Can you work these out from the model? Positions are in its coordinate system, mm. A direction names the side the tool comes from. Coordinates: 2 decimals unless noted, no trailing zeros. Write each loop counter-clockwise with the first axis right and the second up, starting at its lowest first coordinate (ties: lowest second). Pieces come first, ordered by that corner, then holes. Notation, with made-up numbers: (-24.5, -21) - (32.5, -21) arc R22 cw to (32.5, 15) - close; hole circle Ø7 at (-4, 56). An arc over 180 degrees is marked (long way). Use one line per item in the form item = value. Start each with the question number.
(1) If I drill on probe 1 along Z at (x, y) = (-14, 12); probe 2 along Y at (x, z) = (-35, -5.9); probe 3 along Y at (x, z) = (-23, -4), over which ranges is the centre line in solid material (lowest first)? Write a range as from..to.
(2) For pin 1 Ø2.5 at (x, y) = (45.89, 14.18) entering from -Z; pin 2 Ø2.5 at (x, y) = (74.11, 14.18) entering from +Z; pin 3 Ø3 at (y, z) = (2, 3) entering from +X; pin 4 Ø4.5 at (x, z) = (34, 1) entering from -Y, each with a flat end and sliding along its axis, tell me the tip position at first contact or that it passes through.
(3) On a 3-axis mill with a long thin cutter (end or side, diameter ignored), from which of +Z, -Z, +X, -X, +Y, -Y can I reach the whole of each face in a straight line? I mean faces 1 (the face through (1, -15, 5)), 2 (the face through (50.5, 0, 3)), 3 (the face through (-45, 0, -6)). Say none if no direction works.
(4) If we section it at B-B on x = -42: Please give me the cut outline in (y, z).
(5) If we section it at A-A on x = 41: Please give me the cut outline in (y, z), then the cut area to 3 significant figures.
(6) Thinking about a two-plate mould opening in Z: for faces 4 (the face through (18.38, 8.25, -5.65)), 5 (the face through (16, 5.072, 0)), which applies, pulls with the +Z half, pulls with the -Z half, needs draft (parallel to the pull), parting line crosses it, or undercut?
```python
from build123d import *

# Parameters (mm, degrees)
EXTRUDE_1_DEPTH          = 60
EXTRUDE_1_DEPTH_BACK     = 70
EXTRUDE_2_DEPTH          = 7.5
EXTRUDE_2_DEPTH_BACK     = 7.5
SKETCH_2_R               = 27
SKETCH_2_R_2             = 23.5
CUT_EXTRUDE_1_DEPTH      = 7.5
CUT_EXTRUDE_1_DEPTH_BACK = 7.5
SKETCH_3_R               = 24.5
SKETCH_4_R               = 24.5
EXTRUDE_3_DEPTH          = 3
EXTRUDE_4_DEPTH          = 2.58
SKETCH_6_R               = 1
CUT_EXTRUDE_2_DEPTH      = 3
SKETCH_7_R               = 1.5
CUT_EXTRUDE_3_DEPTH      = 5.58
CUT_EXTRUDE_4_DEPTH      = 97
CUT_EXTRUDE_5_DEPTH      = 1
CUT_EXTRUDE_5_DEPTH_BACK = 15
CUT_EXTRUDE_6_DEPTH      = 92.401586419
CUT_EXTRUDE_6_DEPTH_BACK = 7.5
SKETCH_10_R              = 2.5
EXTRUDE_6_DEPTH          = 4
EXTRUDE_6_DEPTH_BACK     = 4
EXTRUDE_7_DEPTH          = 4
EXTRUDE_7_DEPTH_BACK     = 4


with BuildPart() as part:
    # Sketch 1 → Extrude 1 (new, two sides: drawn at the far end of the back side and taken through both)
    with BuildSketch(Plane(origin=(0, 0, 0), x_dir=(0, 0, -1), z_dir=(1, 0, 0)).offset(-EXTRUDE_1_DEPTH_BACK)):
        Polygon((7.5, 0), (7.5, 15), (-7.5, 15), (-7.5, -15), (7.5, -15), align=None)
    extrude(amount=EXTRUDE_1_DEPTH + EXTRUDE_1_DEPTH_BACK)

    # Sketch 2 → Extrude 2 (add, two sides: drawn at the far end of the back side and taken through both)
    with BuildSketch(Plane.XY.offset(-EXTRUDE_2_DEPTH_BACK)):
        with Locations((60, 0)):
            Circle(SKETCH_2_R)
        with Locations((60, 0)):
            Circle(SKETCH_2_R_2, mode=Mode.SUBTRACT)
    extrude(amount=EXTRUDE_2_DEPTH + EXTRUDE_2_DEPTH_BACK)

    # Sketch 3 → Cut-Extrude 1 (cut, two sides: drawn at the far end of the back side and taken through both)
    with BuildSketch(Plane.XY.offset(-CUT_EXTRUDE_1_DEPTH_BACK)):
        with Locations((60, 0)):
            Circle(SKETCH_3_R)
    extrude(amount=CUT_EXTRUDE_1_DEPTH + CUT_EXTRUDE_1_DEPTH_BACK, mode=Mode.SUBTRACT)

    # Sketch 4 → Extrude 3 (add)
    with BuildSketch(Plane.XY.offset(7.5)):
        with Locations((60, 0)):
            Circle(SKETCH_4_R)
    extrude(amount=-EXTRUDE_3_DEPTH)

    # Sketch 5 → Extrude 4 (add)
    with BuildSketch(Plane(origin=(0, 0, 4.5), x_dir=(-1, 0, 0), z_dir=(0, 0, -1))):
        Polygon((-36.5, 0), (-36.5, 4), (-40.5, 4), (-45.5, 4), (-50.5, 4), (-50.5, 0), (-50.5, -4), (-36.5, -4), align=None)
    extrude(amount=EXTRUDE_4_DEPTH)

    # Sketch 6 → Cut-Extrude 2 (cut)
    with BuildSketch(Plane(origin=(0, 0, 4.5), x_dir=(-1, 0, 0), z_dir=(0, 0, -1))):
        with Locations((-60, 20.5)):
            Circle(SKETCH_6_R)
        with Locations((-60, -20.5)):
            Circle(SKETCH_6_R)
        with Locations((-45.894936823, 14.179111142)):
            Circle(SKETCH_6_R)
        with Locations(Location((-74.105063177, 14.179111142, 0), (0, 0, 180))):
            Circle(SKETCH_6_R)
        with Locations((-74.105063177, -14.179111142)):
            Circle(SKETCH_6_R)
        with Locations(Location((-45.894936823, -14.179111142, 0), (0, 0, 180))):
            Circle(SKETCH_6_R)
    extrude(amount=-CUT_EXTRUDE_2_DEPTH, mode=Mode.SUBTRACT)

    # Sketch 7 → Cut-Extrude 3 (cut)
    with BuildSketch(Plane(origin=(0, 0, 1.92), x_dir=(-1, 0, 0), z_dir=(0, 0, -1))):
        with Locations((-47.5, 0)):
            Circle(SKETCH_7_R)
        with Locations((-41, 0)):
            Circle(SKETCH_7_R)
    extrude(amount=-CUT_EXTRUDE_3_DEPTH, mode=Mode.SUBTRACT)

    # Sketch 8 → Cut-Extrude 4 (cut)
    with BuildSketch(Plane.ZY.offset(70)):
        Polygon((0, 15), (-3.75, 15), (-3.75, -15), (3.75, -15), (3.75, 15), align=None)
    extrude(amount=-CUT_EXTRUDE_4_DEPTH, mode=Mode.SUBTRACT)

    # Sketch 9 → Cut-Extrude 5 (cut, two sides: drawn at the far end of the back side and taken through both)
    with BuildSketch(Plane(origin=(36.5, 0, 0), x_dir=(0, 0, -1), z_dir=(1, 0, 0)).offset(-CUT_EXTRUDE_5_DEPTH_BACK)):
        Polygon((3.75, -9.1), (-4.5, -9.1), (-4.5, 9.1), (3.75, 9.1), (3.75, 0), align=None)
    extrude(amount=CUT_EXTRUDE_5_DEPTH + CUT_EXTRUDE_5_DEPTH_BACK, mode=Mode.SUBTRACT)

    # Sketch 10 → Cut-Extrude 6 (cut, two sides: drawn at the far end of the back side and taken through both)
    with BuildSketch(Plane.XY.offset(-CUT_EXTRUDE_6_DEPTH_BACK)):
        with BuildLine():
            Line((-60, 10), (-35, 15))
            Line((-35, 15), (-70, 15))
            Line((-70, 15), (-70, 8.3e-08))
            ThreePointArc((-70, 8.3e-08), (-67.071067782, 7.071067841), (-60, 10))
        make_face()
        with BuildLine():
            ThreePointArc((-60, -10), (-67.071067841, -7.071067782), (-70, 8.3e-08))
            Line((-70, 8.3e-08), (-70, -15))
            Line((-70, -15), (-35, -15))
            Line((-35, -15), (-60, -10))
        make_face()
        with Locations(Location((-60, 0, 0), (0, 0, 180))):
            Circle(SKETCH_10_R)
        with BuildLine():
            Line((-53.381882594, -6.370057829), (-47.910318504, -7.502760494))
            ThreePointArc((-47.910318504, -7.502760494), (-44.955257563, -6.500012961), (-44.393173811, -3.430493514))
            ThreePointArc((-44.393173811, -3.430493514), (-45, 0), (-44.393173811, 3.430493514))
            ThreePointArc((-44.393173811, 3.430493514), (-44.955257563, 6.500012961), (-47.910318504, 7.502760494))
            Line((-47.910318504, 7.502760494), (-53.381882594, 6.370057829))
            ThreePointArc((-53.381882594, 6.370057829), (-55.459731516, 4.768530579), (-55.483580368, 2.145216472))
            ThreePointArc((-55.483580368, 2.145216472), (-55, 0), (-55.483580368, -2.145216472))
            ThreePointArc((-55.483580368, -2.145216472), (-55.459731516, -4.768530579), (-53.381882594, -6.370057829))
        make_face()
        with Locations(Location((-35, 0, 0), (0, 0, 180))):
            Circle(SKETCH_10_R)
        with BuildLine():
            Line((-23.900962122, -10), (-21.539858023, -10))
            ThreePointArc((-21.539858023, -10), (-20.162567137, -9.674865726), (-19.076085186, -8.768113582))
            Line((-19.076085186, -8.768113582), (-8.695659254, 5.072454327))
            ThreePointArc((-8.695659254, 5.072454327), (-8.404850319, 8.29757484), (-11.159432091, 10))
            Line((-11.159432091, 10), (-23.900962122, 10))
            ThreePointArc((-23.900962122, 10), (-26.593808125, 8.414683944), (-26.514312819, 5.290851828))
            ThreePointArc((-26.514312819, 5.290851828), (-25, 0), (-26.514312819, -5.290851828))
            ThreePointArc((-26.514312819, -5.290851828), (-26.593808125, -8.414683944), (-23.900962122, -10))
        make_face()
        with BuildLine():
            Line((-0.923914814, 8.768113582), (-11.304340746, -5.072454327))
            ThreePointArc((-11.304340746, -5.072454327), (-11.595149681, -8.29757484), (-8.840567909, -10))
            Line((-8.840567909, -10), (5, -10))
            Line((5, -10), (5, 10))
            Line((5, 10), (1.539858023, 10))
            ThreePointArc((1.539858023, 10), (0.162567137, 9.674865726), (-0.923914814, 8.768113582))
        make_face()
        with BuildLine():
            Line((5, 10), (5, -10))
            Line((5, -10), (18.840567909, -10))
            ThreePointArc((18.840567909, -10), (21.595149681, -8.29757484), (21.304340746, -5.072454327))
            Line((21.304340746, -5.072454327), (10.923914814, 8.768113582))
            ThreePointArc((10.923914814, 8.768113582), (9.837432863, 9.674865726), (8.460141977, 10))
            Line((8.460141977, 10), (5, 10))
        make_face()
        with BuildLine():
            ThreePointArc((31.715728753, 10), (30, 0), (31.715728753, -10))
            Line((31.715728753, -10), (31.539858023, -10))
            ThreePointArc((31.539858023, -10), (30.162567137, -9.674865726), (29.076085186, -8.768113582))
            Line((29.076085186, -8.768113582), (18.695659254, 5.072454327))
            ThreePointArc((18.695659254, 5.072454327), (18.404850319, 8.29757484), (21.159432091, 10))
            Line((21.159432091, 10), (31.715728753, 10))
        make_face()
    extrude(amount=CUT_EXTRUDE_6_DEPTH + CUT_EXTRUDE_6_DEPTH_BACK, mode=Mode.SUBTRACT)

    # Sketch 12 → Extrude 6 (add, two sides: drawn at the far end of the back side and taken through both)
    with BuildSketch(Plane.XY.offset(-EXTRUDE_6_DEPTH_BACK)):
        Polygon((26.304340746, -5.072454327), (18.695659254, 5.072454327), (13.695659254, 5.072454327), (21.304340746, -5.072454327), (24.981384918, -9.975179891), (29.981384918, -9.975179891), align=None)
        with BuildLine():
            ThreePointArc((-8.695659254, 5.072454327), (-8.079716045, 6.920283955), (-8.695659254, 8.768113582))
            Line((-8.695659254, 8.768113582), (-0.923914814, 8.768113582))
            Line((-0.923914814, 8.768113582), (-3.362056873, 5.517257503))
            Line((-3.362056873, 5.517257503), (-13.88587222, -1.847829627))
            Line((-13.88587222, -1.847829627), (-8.695659254, 5.072454327))
        make_face()
    extrude(amount=EXTRUDE_6_DEPTH + EXTRUDE_6_DEPTH_BACK)

    # Sketch 11 → Extrude 7 (add, two sides: drawn at the far end of the back side and taken through both)
    with BuildSketch(Plane.XY.offset(-EXTRUDE_7_DEPTH_BACK)):
        with BuildLine():
            Line((-65, 8.660254038), (-63.75, 6.495190528))
            ThreePointArc((-63.75, 6.495190528), (-61.941142838, 7.244443697), (-60, 7.5))
            Line((-60, 7.5), (-34.519230769, 12.596153846))
            Line((-34.519230769, 12.596153846), (32.772497208, 12.596153846))
            ThreePointArc((32.772497208, 12.596153846), (33.368731111, 13.812151076), (34.019237886, 15))
            Line((34.019237886, 15), (-35, 15))
            Line((-35, 15), (-60, 10))
            ThreePointArc((-60, 10), (-62.588190451, 9.659258263), (-65, 8.660254038))
        make_face()
    extrude(amount=EXTRUDE_7_DEPTH + EXTRUDE_7_DEPTH_BACK)


solid = part.part
```
Reported:
q1.probe_1 = -7.5..-3.75, 3.75..7.5
q1.probe_2 = -15..-2.5, 2.5..15
q1.probe_3 = -15..-10, 10..15
q2.pin_1 = 4.5
q2.pin_2 = 7.5
q2.pin_3 = 87
q2.pin_4 = -15
q3.face_1 = +Z, -Z, -X, -Y
q3.face_2 = -Z
q3.face_3 = +Z, -Z
q4.outline = (-13.6, -7.5) - (13.6, -7.5) - (13.6, 7.5) - (-13.6, 7.5) - (-13.6, 3.75) - (11.1, 3.75) - (11.1, -3.75) - (-13.6, -3.75) - close
q5.outline = (-19.18, -7.5) - (-15.47, -7.5) - (-15.47, 4.5) - (-4, 4.5) - (-4, 1.92) - (-1.5, 1.92) - (-1.5, 7.5) - (-19.18, 7.5) - close; (1.5, 1.92) - (4, 1.92) - (4, 4.5) - (15.47, 4.5) - (15.47, -7.5) - (19.18, -7.5) - (19.18, 7.5) - (1.5, 7.5) - close
q5.area = 208 mm2
q6.face_4 = needs draft
q6.face_5 = undercut
